```python
from build123d import *

# Parameters (mm, degrees)
F1_DEPTH = 431.8
F2_R     = 27.741248
F3_DEPTH = 51.816
F4_R     = 36.461975
F5_DEPTH = 1447.8


with BuildPart() as f1:
    # F0 (on Front) → F1 (new body)
    with BuildSketch(Plane.XZ):
        Polygon((78.76529, -134.798247), (156.121351, 0.813618), (77.356061, 135.611866), (-78.76529, 134.798247), (-156.121351, -0.813618), (-77.356061, -135.611866), align=None)
    extrude(amount=F1_DEPTH)

    # F2 (on face) → F3 (join)
    with BuildSketch(Plane.XZ.offset(431.8)):
        Circle(F2_R)
    extrude(amount=F3_DEPTH)

    # F4 (on Right) → F5 (join, symmetric)
    with BuildSketch(Plane.YZ):
        with Locations((-200.54774, 0)):
            Circle(F4_R)
    extrude(amount=F5_DEPTH, both=True)


solid = f1.part
```
Work out the finished part from the listing and answer in its coordinate system (mm). A direction names the side the tool comes from. Round coordinates to 2 decimals unless told otherwise and drop trailing zeros. Order: outer loops, then holes, each group sorted by start corner. A loop starts at its lowest first (then second) coordinate and runs counter-clockwise, first axis right, second up.
Q1. A cutting plane is placed at A-A, the plane y = -192.5. Determine the outline of the cut face in (x, z).
Solution:
outline: (-1447.8, -35.56) - (-135.82, -35.56) - (-77.36, -135.61) - (78.77, -134.8) - (135.37, -35.56) - (1447.8, -35.56) - (1447.8, 35.56) - (135.82, 35.56) - (77.36, 135.61) - (-78.77, 134.8) - (-135.37, 35.56) - (-1447.8, 35.56) - close
Q2. A cutting plane is placed at D-D, the plane x = 1103. Determine the outline of the cut face in (y, z).
Solution:
outline: circle Ø72.92 at (-200.55, 0)
Q3. Find the intervals of material crossed by line 1 along Z through (x, y) = (-764.5, -224); line 2 along Y through (x, z) = (-70.5, -28.5); line 3 along Y through (x, z) = (310.5, -1.5), in increasing order.
Solution:
line 1: z = -27.92 to 27.92
line 2: y = -431.8 to 0
line 3: y = -236.98 to -164.12
Q4. A tool of negligible diameter and unlimited length cuts with its end or side. For faces 1 (the flat face through (1447.8, -201, 1)), 2 (the cylindrical face through (-781.8, -227.422, 24.643)), 3 (the cylindrical face through (-22, -457.3, -16.9)), 4 (the cylindrical face through (800.19, -227.422, 24.643)), from which of +Z, -Z, +X, -X, +Y, -Y can it reach the whole face along a straight path? Write none if from no direction.
Solution:
face 1: +Z, -Z, +X, +Y, -Y
face 2: -X
face 3: -Y
face 4: +X
Q5. A cutting plane is placed at C-C, the plane z = 69.5. Determine the outline of the cut face in (x, y).
Solution:
outline: (-116.01, -431.8) - (115.99, -431.8) - (115.99, 0) - (-116.01, 0) - close
Q6. A cutting plane is placed at B-B, the plane x = 0. Determine the outline of the cut face in (y, z).
Solution:
outline: (-483.62, -27.74) - (-431.8, -27.74) - (-431.8, -135.21) - (0, -135.21) - (0, 135.21) - (-431.8, 135.21) - (-431.8, 27.74) - (-483.62, 27.74) - close
Q7. Given pin 1 Ø10 at (y, z) = (-307, -21) entering from -X; pin 2 Ø4 at (y, z) = (-344, 44) entering from -X; pin 3 Ø6 at (y, z) = (-179, -77) entering from +X, each flat-ended and moving along its own axis, determine where each tip first touches the part or whether it passes through.
Solution:
pin 1: stops at x = -147.25
pin 2: stops at x = -131.7
pin 3: stops at x = 113.45
